Design review of the part built by this model. Coordinates are the model's own, in mm. A direction names the side the tool comes from. Give positions to 0.01 mm unless a question says otherwise; leave off trailing zeros. Write each loop counter-clockwise with the first axis right and the second up, starting at its lowest first coordinate (ties: lowest second). Pieces come first, ordered by that corner, then holes. Notation, with made-up numbers: (48, -30) -> (87, -30) arc R13 cw to (87, -17) -> close; hole circle Ø11 at (-37, 5.25). An arc over 180 degrees is marked (long way). Use CSV: the item, a comma, the result in double quotes.
```python
from build123d import *

# Parameters (mm, degrees)
PAD_DEPTH       = 10
POCKET_DEPTH    = 5
SKETCH002_W     = 0.5
SKETCH002_H     = 0.95
PAD001_DEPTH    = 2
SKETCH005_W     = 10
SKETCH005_H     = 10
POCKET001_DEPTH = 2.251
PAD002_DEPTH    = 1
FILLET_R        = 1


with BuildPart() as part:
    # Sketch → Pad (new body)
    with BuildSketch(Plane.XY):
        with BuildLine():
            ThreePointArc((-1.65, 2.75), (-4.4, 0), (-1.65, -2.75))
            Line((-1.65, -2.75), (1.65, -2.75))
            ThreePointArc((1.65, -2.75), (4.4, 0), (1.65, 2.75))
            Line((1.65, 2.75), (-1.65, 2.75))
        make_face()
    extrude(amount=PAD_DEPTH)

    # Sketch001 → Pocket (cut)
    with BuildSketch(Plane.XY):
        Polygon((-3.25, 1.95), (-3.25, 1.15), (-5.25, 1.15), (-5.25, -1.15), (-3.25, -1.15), (-3.25, -1.95), (3.25, -1.95), (3.25, -1.15), (5.25, -1.15), (5.25, 1.15), (3.25, 1.15), (3.25, 1.95), align=None)
    extrude(amount=POCKET_DEPTH, mode=Mode.SUBTRACT)

    # Sketch002 → Pad001 (join, symmetric)
    with BuildSketch(Plane.XZ):
        with Locations((-0.75, 4.525)):
            Rectangle(SKETCH002_W, SKETCH002_H)
        with Locations((0.75, 4.525)):
            Rectangle(SKETCH002_W, SKETCH002_H)
    extrude(amount=PAD001_DEPTH, both=True)

    # Sketch005 (on DatumPlane) → Pocket001 (cut, through all)
    with BuildSketch(Plane.XY.offset(7.75)):
        Rectangle(SKETCH005_W, SKETCH005_H)
        with BuildLine():
            ThreePointArc((-1.5, 1.35), (-2.85, 0), (-1.5, -1.35))
            Line((-1.5, -1.35), (1.5, -1.35))
            ThreePointArc((1.5, -1.35), (2.85, 0), (1.5, 1.35))
            Line((1.5, 1.35), (-1.5, 1.35))
        make_face(mode=Mode.SUBTRACT)
    extrude(amount=POCKET001_DEPTH, mode=Mode.SUBTRACT)

    # Sketch006 → Pad002 (join)
    with BuildSketch(Plane.XY):
        Polygon((-2.714303, -2.535697), (-1.5, -3.75), (1.5, -3.75), (2.714303, -2.535697), align=None)
    pad002 = extrude(amount=PAD002_DEPTH)

    # Mirrored: Pad002 across XZ
    add(pad002.mirror(Plane.XZ))

    # Fillet
    fillet_edges = [part.edges().sort_by_distance(p)[0] for p in [
        (0, -1.35, 10),
        (2.85, 0, 10),
        (0, 1.35, 10),
        (-2.85, 0, 10),
    ]]
    fillet(fillet_edges, radius=FILLET_R)


solid = part.part
```
(1) Clearance check with flat-ended pins moving along their axes: pin 1 (1 mm diameter, centred on x = 3.5, z = 3.5, fed in from -Y); pin 2 (1.3 mm diameter, centred on x = 0, y = -3.5, fed in from +Z); pin 3 (1 mm diameter, centred on x = 2.5, y = -0.5, fed in from +Z). State where each tip first meets the part, or that it passes through.
Established:
pin 1,"stops at y = -2.4"
pin 2,"stops at z = 1"
pin 3,"stops at z = 9.96"
(2) For line 1 along Z through (x, y) = (0.25, -2); line 2 along Y through (x, z) = (2, 0.5); line 3 along Y through (x, z) = (-1, 3.25), list the stretches that pass through material, from the lowest coordinate up. Write a range as [from, to].
Established:
line 1,"z = [0, 7.75]"
line 2,"y = [-3.25, -1.95], [1.95, 3.25]"
line 3,"y = [-2.75, -1.95], [1.95, 2.75]"
(3) Take a section at B-B (x = -1.25). Write out the cut boundary in (y, z), then the cut area to 3 significant figures.
Established:
outline,"(-3.75, 0) -> (-1.95, 0) -> (-1.95, 5) -> (1.95, 5) -> (1.95, 0) -> (3.75, 0) -> (3.75, 1) -> (2.75, 1) -> (2.75, 7.75) -> (1.35, 7.75) -> (1.35, 9) arc R1 ccw to (0.35, 10) -> (-0.35, 10) arc R1 ccw to (-1.35, 9) -> (-1.35, 7.75) -> (-2.75, 7.75) -> (-2.75, 1) -> (-3.75, 1) -> close"
area,"30.8 mm2"
(4) Take a section at D-D (y = 3). Write out the cut boundary in (x, z).
Established:
outline,"(-2.25, 0) -> (2.25, 0) -> (2.25, 1) -> (-2.25, 1) -> close"
(5) Take a section at C-C (z = 7.5). Write out the cut boundary in (x, y).
Established:
outline,"(-1.65, -2.75) -> (1.65, -2.75) arc R2.75 ccw to (1.65, 2.75) -> (-1.65, 2.75) arc R2.75 ccw to start"
(6) Tool access review of faces 4 (the face through (4.4, -0.1, 5.5)), 5 (the face through (0, 2.75, 4)), 6 (the face through (0, 0, 5)), 7 (the face through (-2.85, 0.03, 8.37)), 8 (the face through (0, -2.75, 4)): name each direction out of +Z, -Z, +X, -X, +Y, -Y from which nothing blocks a thin tool from reaching the whole face with its end or side.
Established:
face 4,"+Z, +X"
face 5,"+Z, +X, -X, +Y"
face 6,"-Z"
face 7,"+Z, -X"
face 8,"+Z, +X, -X, -Y"
(7) Take a section at A-A (z = 3.75). Write out the cut boundary in (x, y).
Established:
outline,"(-4.15, -1.15) arc R2.75 ccw to (-1.65, -2.75) -> (1.65, -2.75) arc R2.75 ccw to (4.15, -1.15) -> (3.25, -1.15) -> (3.25, -1.95) -> (-3.25, -1.95) -> (-3.25, -1.15) -> close; (-4.15, 1.15) -> (-3.25, 1.15) -> (-3.25, 1.95) -> (3.25, 1.95) -> (3.25, 1.15) -> (4.15, 1.15) arc R2.75 ccw to (1.65, 2.75) -> (-1.65, 2.75) arc R2.75 ccw to start"
(8) Mouldability with a two-part tool opening along Y and no side actions: class faces 1 (the face through (3.7, 1.15, 2.5)), 2 (the face through (-0.021, -1.065, 9.699)), 3 (the face through (0, 1.35, 8)) as +Y half, -Y half, draft (parallel to the pull), parting line (faces both ways), or undercut.
Established:
face 1,"undercut"
face 2,"-Y half"
face 3,"+Y half"
